Part model, mm, in its own coordinate system. A direction names the side the tool comes from. Round coordinates to 2 decimals unless told otherwise and drop trailing zeros. Write each loop counter-clockwise with the first axis right and the second up, starting at its lowest first coordinate (ties: lowest second). Pieces come first, ordered by that corner, then holes. Notation, with made-up numbers: (46.5, 31.5) -> (60.5, 31.5) arc R20 cw to (60.5, 39.5) -> close; hole circle Ø7 at (-33.5, 23). An arc over 180 degrees is marked (long way). Return JSON: item names as keys, results as strings. Group by question number.
```python
from build123d import *

# Parameters (mm, degrees)
F1_DEPTH = 15
F2_SIZE  = 5


with BuildPart() as f1:
    # F0 (on Top) → F1 (new body)
    with BuildSketch(Plane.XY):
        with BuildLine():
            Line((-186.024674, -9.009846), (-179.286195, -11.425942))
            ThreePointArc((-179.286195, -11.425942), (-179.538284, -10.090694), (-179.280339, -8.756566))
            Line((-179.280339, -8.756566), (-215.305157, 4.16021))
            Line((-215.305157, 4.16021), (-187.557676, -13.285381))
            Line((-187.557676, -13.285381), (-186.024674, -9.009846))
        make_face()
        with BuildLine():
            ThreePointArc((-179.280339, -8.756566), (-178.513831, -7.575145), (-177.354514, -6.775599))
            Line((-177.354514, -6.775599), (-184.327177, -4.275535))
            Line((-184.327177, -4.275535), (-182.794174, 0))
            Line((-182.794174, 0), (-215.305157, 4.16021))
            Line((-215.305157, 4.16021), (-179.280339, -8.756566))
        make_face()
        with BuildLine():
            ThreePointArc((-179.286195, -11.425942), (-175.242569, -13.655259), (-172.297879, -10.098635))
            ThreePointArc((-172.297879, -10.098635), (-173.929905, -7.073238), (-177.354514, -6.775599))
            ThreePointArc((-177.354514, -6.775599), (-178.513831, -7.575145), (-179.280339, -8.756566))
            ThreePointArc((-179.280339, -8.756566), (-179.538284, -10.090694), (-179.286195, -11.425942))
        make_face()
    extrude(amount=F1_DEPTH)

    # F2
    f2_edges = [f1.edges().sort_by_distance(p)[0] for p in [
        (-201.431417, -4.562585, 15),
        (-199.049666, 2.080105, 15),
        (-199.049666, 2.080105, 0),
        (-201.431417, -4.562585, 0),
    ]]
    chamfer(f2_edges, length=F2_SIZE)


solid = f1.part
```
Item 1: Wall check: L1, parallel to Z at x = -187.5, y = -10.5; L2, parallel to X at y = -8.75, z = 1.5; L3, parallel to Y at x = -191, z = 9.25. Give the ranges that are in metal, low to high.
Item 2: Which spindle directions (+Z, -Z, +X, -X, +Y, -Y) get a long thin tool onto all of the face, cutting with end or side? Do faces 5 (the face through (-198.82, 2.05, 7.46)), 6 (the face through (-182.7, -10.2, 7.4)). Say none if no direction does.
Item 3: Cut at B-B (z = 9.25). Write the cut outline in (x, y), then the cut area to 3 significant figures.
Item 4: Two-plate mould, pull along Y, no slides. Class faces 1 (the face through (-194.49, -0.5, 11.98)), 2 (the face through (-186.63, -10.7, 7.4)), 3 (the face through (-180.792, -5.543, 7.395)), 4 (the face through (-183.74, -2.64, 7.4)): released by +Y, released by -Y, zero draft, split by the parting line, or undercut.
Item 5: Cut at A-A (y = -12). Write the cut outline in (x, z).
Item 6: Cut at D-D (y = -2.5). Write the cut outline in (x, z), then the cut area to 3 significant figures.
Item 7: Flat gauge pins, fed straight in: P1, Ø1, axis at x = -195, y = 0, coming from the +Z side; P2, Ø8, axis at y = -5, z = 6, coming from the -X side; P3, Ø6, axis at x = -206, z = 8.5, coming from the -Y side. Where does each tip first touch, or does it go through?
Item 8: Cut at C-C (x = -190). Write the cut outline in (y, z).
Checks:
{
 "1": {"L1": "z = 2.61 to 12.39", "L2": "x = -188.2 to -172.56", "L3": "y = -11.12 to 1.05"},
 "2": {"face 5": "+Z, -Z, +X, +Y", "face 6": "+Z, -Z, -Y"},
 "3": {"outline": "(-215.31, 4.16) -> (-187.56, -13.29) -> (-186.02, -9.01) -> (-179.29, -11.43) arc R3.62 ccw to (-172.3, -10.1) arc R3.62 ccw to (-177.35, -6.78) -> (-184.33, -4.28) -> (-182.79, 0) -> close", "area": "300 mm2"},
 "4": {"face 1": "released by +Y", "face 2": "released by -Y", "face 3": "undercut", "face 4": "undercut"},
 "5": {"outline": "(-189.6, 5) -> (-187.1, 3.67) -> (-187.1, 11.33) -> (-189.6, 10) -> close; (-179, 0) -> (-172.84, 0) -> (-172.84, 15) -> (-179, 15) -> close"},
 "6": {"outline": "(-204.71, 5) -> (-196.73, 0.75) -> (-183.69, 2.41) -> (-183.69, 12.59) -> (-196.73, 14.25) -> (-204.71, 10) -> close", "area": "228 mm2"},
 "7": {"P1": "stops at z = 12.05", "P2": "stops at x = -207.1", "P3": "stops at y = -3.58"},
 "8": {"outline": "(-11.75, 5) -> (-5.84, 0) -> (-4.12, 0) -> (0.92, 5) -> (0.92, 10) -> (-4.12, 15) -> (-5.84, 15) -> (-11.75, 10) -> close"}
}
